from build123d import *

# Parameters (mm, degrees)
BOSS_EXTRUDE1_DEPTH = 12
SKETCH2_R           = 6
BOSS_EXTRUDE2_DEPTH = 12
SKETCH3_R           = 5
CUT_EXTRUDE1_DEPTH  = 12
FILLET1_R           = 0.75
FILLET2_R           = 0.75
FILLET3_R           = 0.75
FILLET4_R           = 0.75


with BuildPart() as part:
    # Sketch1 → Boss-Extrude1 (new body)
    with BuildSketch(Plane.XY):
        with BuildLine():
            Line((-1, 9.949874371), (-2, 10.816653826))
            ThreePointArc((-2, 10.816653826), (0, 11), (2, 10.816653826))
            Line((2, 10.816653826), (1, 9.949874371))
            Line((1, 9.949874371), (1, 4.898979486))
            ThreePointArc((1, 4.898979486), (1.294095226, 4.829629131), (1.583464339, 4.742640687))
            Line((1.583464339, 4.742640687), (4.108911782, 9.11684397))
            Line((4.108911782, 9.11684397), (3.676276106, 10.367496998))
            ThreePointArc((3.676276106, 10.367496998), (5.5, 9.526279442), (7.140377721, 8.367496998))
            Line((7.140377721, 8.367496998), (5.840962589, 8.11684397))
            Line((5.840962589, 8.11684397), (3.315515147, 3.742640687))
            ThreePointArc((3.315515147, 3.742640687), (3.535533906, 3.535533906), (3.742640687, 3.315515147))
            Line((3.742640687, 3.315515147), (8.11684397, 5.840962589))
            Line((8.11684397, 5.840962589), (8.367496998, 7.140377721))
            ThreePointArc((8.367496998, 7.140377721), (9.526279442, 5.5), (10.367496998, 3.676276106))
            Line((10.367496998, 3.676276106), (9.11684397, 4.108911782))
            Line((9.11684397, 4.108911782), (4.742640687, 1.583464339))
            ThreePointArc((4.742640687, 1.583464339), (4.829629131, 1.294095226), (4.898979486, 1))
            Line((4.898979486, 1), (9.949874371, 1))
            Line((9.949874371, 1), (10.816653826, 2))
            ThreePointArc((10.816653826, 2), (11, 0), (10.816653826, -2))
            Line((10.816653826, -2), (9.949874371, -1))
            Line((9.949874371, -1), (4.898979486, -1))
            ThreePointArc((4.898979486, -1), (4.829629131, -1.294095226), (4.742640687, -1.583464339))
            Line((4.742640687, -1.583464339), (9.11684397, -4.108911782))
            Line((9.11684397, -4.108911782), (10.367496998, -3.676276106))
            ThreePointArc((10.367496998, -3.676276106), (9.526279442, -5.5), (8.367496998, -7.140377721))
            Line((8.367496998, -7.140377721), (8.11684397, -5.840962589))
            Line((8.11684397, -5.840962589), (3.742640687, -3.315515147))
            ThreePointArc((3.742640687, -3.315515147), (3.535533906, -3.535533906), (3.315515147, -3.742640687))
            Line((3.315515147, -3.742640687), (5.840962589, -8.11684397))
            Line((5.840962589, -8.11684397), (7.140377721, -8.367496998))
            ThreePointArc((7.140377721, -8.367496998), (5.5, -9.526279442), (3.676276106, -10.367496998))
            Line((3.676276106, -10.367496998), (4.108911782, -9.11684397))
            Line((4.108911782, -9.11684397), (1.583464339, -4.742640687))
            ThreePointArc((1.583464339, -4.742640687), (1.294095226, -4.829629131), (1, -4.898979486))
            Line((1, -4.898979486), (1, -9.949874371))
            Line((1, -9.949874371), (2, -10.816653826))
            ThreePointArc((2, -10.816653826), (0, -11), (-2, -10.816653826))
            Line((-2, -10.816653826), (-1, -9.949874371))
            Line((-1, -9.949874371), (-1, -4.898979486))
            ThreePointArc((-1, -4.898979486), (-1.294095226, -4.829629131), (-1.583464339, -4.742640687))
            Line((-1.583464339, -4.742640687), (-4.108911782, -9.11684397))
            Line((-4.108911782, -9.11684397), (-3.676276106, -10.367496998))
            ThreePointArc((-3.676276106, -10.367496998), (-5.5, -9.526279442), (-7.140377721, -8.367496998))
            Line((-7.140377721, -8.367496998), (-5.840962589, -8.11684397))
            Line((-5.840962589, -8.11684397), (-3.315515147, -3.742640687))
            ThreePointArc((-3.315515147, -3.742640687), (-3.535533906, -3.535533906), (-3.742640687, -3.315515147))
            Line((-3.742640687, -3.315515147), (-8.11684397, -5.840962589))
            Line((-8.11684397, -5.840962589), (-8.367496998, -7.140377721))
            ThreePointArc((-8.367496998, -7.140377721), (-9.526279442, -5.5), (-10.367496998, -3.676276106))
            Line((-10.367496998, -3.676276106), (-9.11684397, -4.108911782))
            Line((-9.11684397, -4.108911782), (-4.742640687, -1.583464339))
            ThreePointArc((-4.742640687, -1.583464339), (-4.829629131, -1.294095226), (-4.898979486, -1))
            Line((-4.898979486, -1), (-9.949874371, -1))
            Line((-9.949874371, -1), (-10.816653826, -2))
            ThreePointArc((-10.816653826, -2), (-11, 0), (-10.816653826, 2))
            Line((-10.816653826, 2), (-9.949874371, 1))
            Line((-9.949874371, 1), (-4.898979486, 1))
            ThreePointArc((-4.898979486, 1), (-4.829629131, 1.294095226), (-4.742640687, 1.583464339))
            Line((-4.742640687, 1.583464339), (-9.11684397, 4.108911782))
            Line((-9.11684397, 4.108911782), (-10.367496998, 3.676276106))
            ThreePointArc((-10.367496998, 3.676276106), (-9.526279442, 5.5), (-8.367496998, 7.140377721))
            Line((-8.367496998, 7.140377721), (-8.11684397, 5.840962589))
            Line((-8.11684397, 5.840962589), (-3.742640687, 3.315515147))
            ThreePointArc((-3.742640687, 3.315515147), (-3.535533906, 3.535533906), (-3.315515147, 3.742640687))
            Line((-3.315515147, 3.742640687), (-5.840962589, 8.11684397))
            Line((-5.840962589, 8.11684397), (-7.140377721, 8.367496998))
            ThreePointArc((-7.140377721, 8.367496998), (-5.5, 9.526279442), (-3.676276106, 10.367496998))
            Line((-3.676276106, 10.367496998), (-4.108911782, 9.11684397))
            Line((-4.108911782, 9.11684397), (-1.583464339, 4.742640687))
            ThreePointArc((-1.583464339, 4.742640687), (-1.294095226, 4.829629131), (-1, 4.898979486))
            Line((-1, 4.898979486), (-1, 9.949874371))
        make_face()
    extrude(amount=BOSS_EXTRUDE1_DEPTH)

    # Sketch2 → Boss-Extrude2 (add)
    with BuildSketch(Plane.XY.offset(12)):
        Circle(SKETCH2_R)
    extrude(amount=-BOSS_EXTRUDE2_DEPTH)

    # Sketch3 → Cut-Extrude1 (cut)
    with BuildSketch(Plane.XY.offset(12)):
        Circle(SKETCH3_R)
    extrude(amount=-CUT_EXTRUDE1_DEPTH, mode=Mode.SUBTRACT)

    # Fillet1
    fillet1_edges = [part.edges().sort_by_distance(p)[0] for p in [
        (-4.623475383, 3.824065295, 6),
    ]]
    fillet(fillet1_edges, radius=FILLET1_R)

    # Fillet2
    # the kernel refuses this fillet: 0.75 mm, written as the material it adds along each edge
    with BuildSketch(Plane(origin=(-3.824065295, 4.623475383, 0), x_dir=(-0.7395125518358552, -0.6731427676780178, 0), z_dir=(0, 0, 1))) as fillet2_piece_1:
        with BuildLine():
            CenterArc((0.604168803, -0.749157497), FILLET2_R, 92.716022766, 74.973886241)
            Line((-0.128587227, -0.589255651), (0, 0))
            ThreePointArc((0, 0), (0.284314731, -0.006740024), (0.568629461, 0))
        make_face()
    extrude(amount=12)

    # Fillet3
    fillet3_edges = [part.edges().sort_by_distance(p)[0] for p in [
        (3.824065295, 4.623475383, 6),
        (1, 5.916079783, 6),
        (-2.092014488, 5.623475383, 6),
        (-5.916079783, 1, 6),
        (-5.623475383, -2.092014488, 6),
        (-3.824065295, -4.623475383, 6),
        (-1, -5.916079783, 6),
        (2.092014488, -5.623475383, 6),
        (4.623475383, -3.824065295, 6),
        (5.916079783, -1, 6),
        (5.623475383, 2.092014488, 6),
    ]]
    fillet(fillet3_edges, radius=FILLET3_R)

    # Fillet4
    # the kernel refuses this fillet: 0.75 mm, written as the material it adds along each edge
    with BuildSketch(Plane(origin=(-5.916079783, -1, 0), x_dir=(-1, 0, 0), z_dir=(0, 0, 1)), Plane(origin=(-4.623475383, -3.824065295, 0), x_dir=(-0.8660254037844433, -0.4999999999999918, 0), z_dir=(0, 0, 1)), Plane(origin=(-2.092014488, -5.623475383, 0), x_dir=(-0.5000000000000068, -0.8660254037844348, 0), z_dir=(0, 0, 1)), Plane(origin=(1, -5.916079783, 0), x_dir=(0, -1, 0), z_dir=(0, 0, 1)), Plane(origin=(-5.623475383, 2.092014488, 0), x_dir=(-0.8660254037844328, 0.5000000000000101, 0), z_dir=(0, 0, 1))) as fillet4_piece_1:
        with BuildLine():
            CenterArc((0.603099347, 0.75), FILLET4_R, 195.444398539, 74.555601461)
            Line((-0.119817654, 0.550272663), (-0.134275994, 0.546278116))
            ThreePointArc((-0.134275994, 0.546278116), (-0.068105699, 0.273351526), (-0.014790199, -0.0025))
            Line((-0.014790199, -0.0025), (0, -0.015))
            Line((0, -0.015), (0.603099347, -0.015))
            Line((0.603099347, -0.015), (0.603099347, 0))
        make_face()
    extrude(amount=12)
    with BuildSketch(Plane(origin=(3.824065295, -4.623475383, 0), x_dir=(0.7398192740207736, 0.6728056493426431, 0), z_dir=(0, 0, 1)), Plane(origin=(5.623475383, -2.092014488, 0), x_dir=(0.30429946084002696, 0.9525764211508013, 0), z_dir=(0, 0, 1)), Plane(origin=(5.916079783, 1, 0), x_dir=(-0.21275714713002825, 0.9771051101826719, 0), z_dir=(0, 0, 1)), Plane(origin=(4.623475383, 3.824065295, 0), x_dir=(-0.6728056493426434, 0.7398192740207732, 0), z_dir=(0, 0, 1)), Plane(origin=(2.092014488, 5.623475383, 0), x_dir=(-0.9525764211508011, 0.30429946084002774, 0), z_dir=(0, 0, 1)), Plane(origin=(-1, 5.916079783, 0), x_dir=(-0.9771051101826725, -0.21275714713002564, 0), z_dir=(0, 0, 1))) as fillet4_piece_2:
        with BuildLine():
            CenterArc((0.604515136, -0.748859315), FILLET4_R, 93.160421305, 74.555601461)
            Line((-0.128313697, -0.589291454), (-0.142970273, -0.586100097))
            Line((-0.142970273, -0.586100097), (-0.014656577, 0.003191357))
            Line((-0.014656577, 0.003191357), (0.000703958, 0.014983472))
            ThreePointArc((0.000703958, 0.014983472), (0.281583147, 0.008388935), (0.562339316, 0.014977186))
            Line((0.562339316, 0.014977186), (0.563166293, 0))
        make_face()
    extrude(amount=12)


solid = part.part
Read the model definition and answer for the solid it produces. Units are mm, in the model's axes. A direction names the side the tool comes from. Round coordinates to 2 decimals unless told otherwise and drop trailing zeros. Loops run counter-clockwise (first coordinate to the right, second up) from the corner with the lowest first, then second, coordinate; pieces in that order, holes last.
Q1. Consider probe 1 along Y at (x, z) = (0, 8.5); probe 2 along X at (y, z) = (9.5, 3.5); probe 3 along X at (y, z) = (10, 9.5). Determine where each line is inside the solid, lowest interval first.
Q2. Which of the six approach directions +Z, -Z, +X, -X, +Y, -Y give full straight-line access (tool end or side, diameter ignored) to faces 4 (the face through (1, 8, 6)), 5 (the face through (-11, 0, 6)), 6 (the face through (-8.244, 6.5, 5.916))?
Q3. Determine the mould class of faces 1 (the face through (9.54, -5.48, 5.92)), 2 (the face through (-5.826, 2.027, 5.916)), 3 (the face through (4, 4, 0)) for opening direction X: released by +X, released by -X, zero draft, split by the parting line, or undercut.
Q4. Section D-D on x = 7.5 is taken. Write down the section's boundary in (y, z), and give its area (3 significant figures).
Q5. Section A-A on y = 0 is taken. Write down the section's boundary in (x, z).
Q6. Each of these flat-tipped pins is pushed along its axis until it touches: pin 1 (9 mm diameter, centred on x = 0, y = 0, fed in from +Z); pin 2 (4 mm diameter, centred on x = -5.5, y = -7, fed in from +Z); pin 3 (2.5 mm diameter, centred on x = -8.5, z = 8, fed in from -Y); pin 4 (1.5 mm diameter, centred on y = 1.5, z = 2, fed in from -X). Where does it stop, or does it pass through?
Q7. Section C-C on y = -7.75 is taken. Write down the section's boundary in (x, z).
Output:
1. probe 1: y = -11 to -5, 5 to 11
1. probe 2: x = -5.55 to -3.98, -1 to 1, 3.98 to 5.55
1. probe 3: x = -4.58 to -3.8, -1.06 to 1.06, 3.8 to 4.58
2. face 4: +Z, -Z
2. face 5: +Z, -Z, -X
2. face 6: +Z, -Z, +Y
3. face 1: released by +X
3. face 2: undercut
3. face 3: zero draft
4. outline: (-5.48, 0) - (-3.18, 0) - (-3.18, 12) - (-5.48, 12) - close; (-1, 0) - (1, 0) - (1, 12) - (-1, 12) - close; (3.18, 0) - (5.48, 0) - (5.48, 12) - (3.18, 12) - close
4. area: 79.4 mm2
5. outline: (-11, 0) - (-5, 0) - (-5, 12) - (-11, 12) - close; (5, 0) - (11, 0) - (11, 12) - (5, 12) - close
6. pin 1: passes through
6. pin 2: stops at z = 12
6. pin 3: stops at y = -7.14
6. pin 4: stops at x = -10.97
7. outline: (-5.63, 0) - (-3.32, 0) - (-3.32, 12) - (-5.63, 12) - close; (-1, 0) - (1, 0) - (1, 12) - (-1, 12) - close; (3.32, 0) - (5.63, 0) - (5.63, 12) - (3.32, 12) - close
